Input: dimensioned drawing with shaded views. Units: mm. Origin: part minimum x, y, z. A direction names the side the tool comes from. Coordinates: 2 decimals unless noted, no trailing zeros. Order: outer loops, then holes, each group sorted by start corner. A loop starts at its lowest first (then second) coordinate and runs counter-clockwise, first axis right, second up. Notation, with made-up numbers: M 15.25,63.5 L 60.25,63.5 A13 ccw 60.25,88.5 Z; hole C 73,-12.5 d8. An arc over 180 degrees is marked long. Write item = value, one per line.
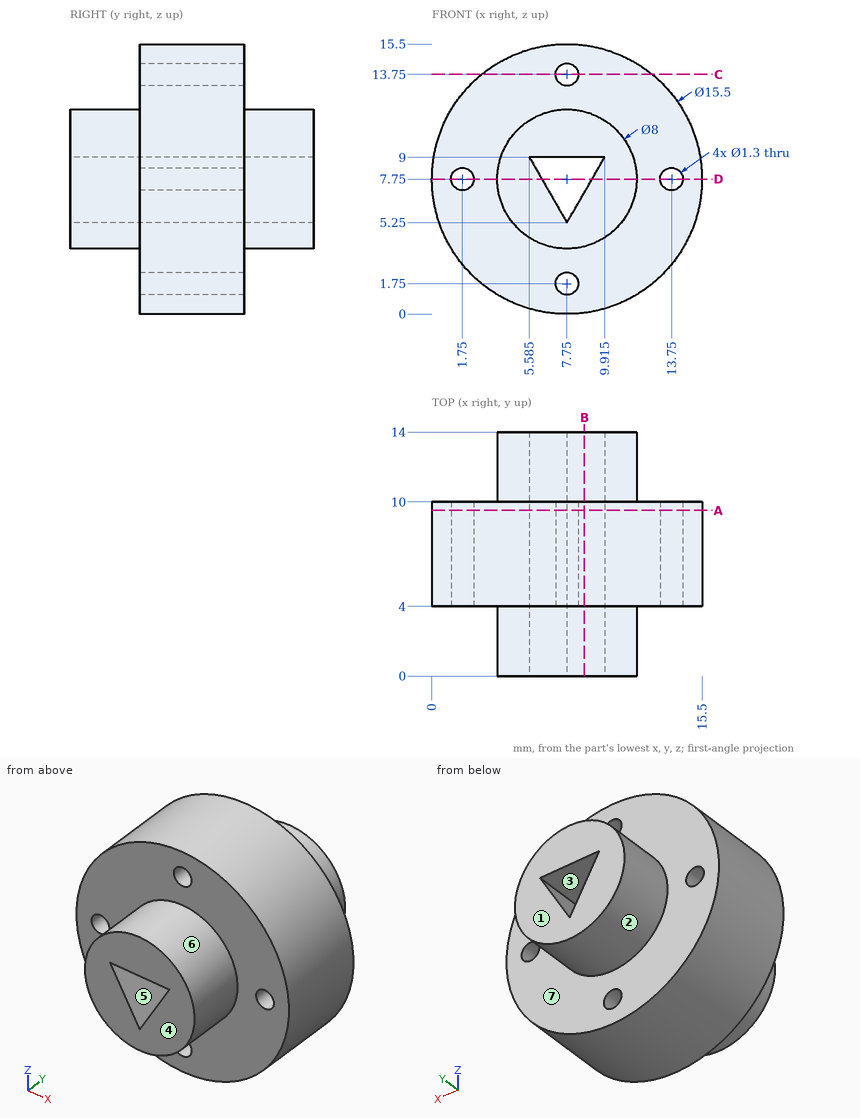
1) Section A-A, the plane y = 9.5. Return loops of the section in (x, z) (3 decimals).
Numbers:
outline = C 7.75,7.75 d15.5; hole C 1.75,7.75 d1.3; hole M 5.585,9 L 7.75,5.25 L 9.915,9 Z; hole C 7.75,1.75 d1.3; hole C 7.75,13.75 d1.3; hole C 13.75,7.75 d1.3
2) Pin query (flat end, axial travel): pin 1 (4 mm diameter, centred on x = 10, y = 7, fed in from +Z); pin 2 (6 mm diameter, centred on y = 11.5, z = 10.5, fed in from -X); pin 3 (6 mm diameter, centred on x = 4.5, y = 4.5, fed in from -Z). Return the tip coordinate at first contact, or that it passes through.
Numbers:
pin_1 = 15.5
pin_2 = 0
pin_3 = 0
3) Line query: L1, parallel to Y at x = 7.5, z = 14.75; L2, parallel to Z at x = 6.75, y = 13; L3, parallel to Z at x = 9, y = 7.75 (1 decimal). Output: solid intervals per line, ascending.
Numbers:
L1 = 4 to 10
L2 = 3.88 to 6.98, 9 to 11.62
L3 = 0.1 to 7.4, 9 to 15.4
4) Mould query, pull axis X, two halves, no side actions, for the marked faces 1, 2 and 3. Classes: pulls with the +X half, pulls with the -X half, needs draft (parallel to the pull), parting line crosses it, or undercut.
Numbers:
face_1 = needs draft
face_2 = parting line crosses it
face_3 = undercut
5) Section C-C, the plane z = 13.75. Return loops of the section in (x, y), and give its area (3 significant figures).
Numbers:
outline = M 2.84,4 L 7.1,4 L 7.1,10 L 2.84,10 Z; M 8.4,4 L 12.66,4 L 12.66,10 L 8.4,10 Z
area = 51.1 mm²
6) Section D-D, the plane z = 7.75. Return loops of the section in (x, y), and give its area (3 significant figures).
Numbers:
outline = M 0,4 L 1.1,4 L 1.1,10 L 0,10 Z; M 2.4,4 L 3.75,4 L 3.75,0 L 6.31,0 L 6.31,14 L 3.75,14 L 3.75,10 L 2.4,10 Z; M 9.19,0 L 11.75,0 L 11.75,4 L 13.1,4 L 13.1,10 L 11.75,10 L 11.75,14 L 9.19,14 Z; M 14.4,4 L 15.5,4 L 15.5,10 L 14.4,10 Z
area = 101 mm²
7) Set-up query: the marked faces 4, 5, 6 and 7. Return all of +Z, -Z, +X, -X, +Y, -Y with unobstructed straight access to the full face (end or side cutting, diameter ignored); none if empty.
Numbers:
face_4 = +Z, -Z, +X, -X, -Y
face_5 = +Y, -Y
face_6 = -Y
face_7 = +Y
8) Section B-B, the plane x = 8.75. Return loops of the section in (y, z).
Numbers:
outline = M 0,3.88 L 4,3.88 L 4,0.06 L 10,0.06 L 10,3.88 L 14,3.88 L 14,6.98 L 0,6.98 Z; M 0,9 L 14,9 L 14,11.62 L 10,11.62 L 10,15.44 L 4,15.44 L 4,11.62 L 0,11.62 Z
